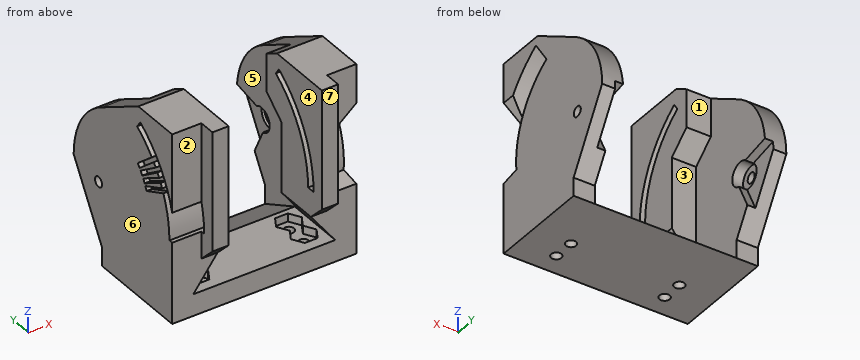
```python
from build123d import *

# Parameters (mm, degrees)
CROQUIS1_W              = 34
CROQUIS1_H              = 19
SALIENTE_EXTRUIR1_DEPTH = 35
CROQUIS2_W              = 26.2
CROQUIS2_H              = 31
CORTAR_EXTRUIR1_DEPTH   = 25
CORTAR_EXTRUIR3_DEPTH   = 26.2
SALIENTE_EXTRUIR2_DEPTH = 34
CROQUIS10_W             = 26.2
CROQUIS10_H             = 25.966324345
CORTAR_EXTRUIR4_DEPTH   = 10
CROQUIS18_R             = 0.95
CORTAR_EXTRUIR11_DEPTH  = 4
CORTAR_EXTRUIR12_DEPTH  = 1.5
CORTAR_EXTRUIR14_START  = -34
CROQUIS21_R             = 0.95
CORTAR_EXTRUIR14_DEPTH  = 34
SALIENTE_EXTRUIR3_DEPTH = 8
CROQUIS25_W             = 3
CROQUIS25_H             = 25
SALIENTE_EXTRUIR4_DEPTH = 3
CROQUIS43_W             = 4.5
CROQUIS43_H             = 12
SALIENTE_EXTRUIR8_DEPTH = 4
CORTAR_EXTRUIR18_DEPTH  = 7.4
CORTAR_EXTRUIR16_START  = -34
CORTAR_EXTRUIR16_DEPTH  = 26.6
CORTAR_EXTRUIR20_START  = -1.5
CORTAR_EXTRUIR20_DEPTH  = 1.5
CORTAR_EXTRUIR21_DEPTH  = 27.7
CORTAR_EXTRUIR22_START  = -34
CORTAR_EXTRUIR22_DEPTH  = 34
CORTAR_EXTRUIR23_DEPTH  = 3
CROQUIS36_R             = 2.2
CORTAR_EXTRUIR24_DEPTH  = 2
CORTAR_EXTRUIR25_START  = 28.2
CROQUIS36_2_R           = 2.2
CORTAR_EXTRUIR25_DEPTH  = 28.2
CORTAR_EXTRUIR26_START  = -34
CORTAR_EXTRUIR26_DEPTH  = 34
CORTAR_EXTRUIR27_DEPTH  = 1
CORTAR_EXTRUIR28_START  = -23.2
CORTAR_EXTRUIR28_DEPTH  = 23.2
CORTAR_EXTRUIR29_DEPTH  = 26.2


with BuildPart() as part:
    # Croquis1 → Saliente-Extruir1 (new body)
    with BuildSketch(Plane.XY):
        with Locations((-31.887263086, 5.12254902)):
            Rectangle(CROQUIS1_W, CROQUIS1_H)
    extrude(amount=SALIENTE_EXTRUIR1_DEPTH)

    # Croquis2 → Cortar-Extruir1 (cut)
    with BuildSketch(Plane.XZ.offset(4.37745098)):
        with Locations((-31.887263086, 19.5)):
            Rectangle(CROQUIS2_W, CROQUIS2_H)
    extrude(amount=-CORTAR_EXTRUIR1_DEPTH, mode=Mode.SUBTRACT)

    # Croquis4 → Cortar-Extruir3 (cut)
    with BuildSketch(Plane.ZY.offset(18.787263086)):
        Polygon((4, 14.62254902), (4, 6.62254902), (0, 14.62254902), align=None)
    extrude(amount=CORTAR_EXTRUIR3_DEPTH, mode=Mode.SUBTRACT)

    # Croquis9 → Saliente-Extruir2 (add)
    with BuildSketch(Plane(origin=(-14.887263086, 0, 0), x_dir=(0, 0, -1), z_dir=(1, 0, 0))):
        with BuildLine():
            Line((-29.315831827, 14.62254902), (-3.349507482, 14.62254902))
            ThreePointArc((-3.349507482, 14.62254902), (-16.332669655, 22.37254902), (-29.315831827, 14.62254902))
        make_face()
    extrude(amount=-SALIENTE_EXTRUIR2_DEPTH)

    # Croquis10 → Cortar-Extruir4 (cut)
    with BuildSketch(Plane.XZ.offset(-14.62254902)):
        with Locations((-31.887263086, 16.332669655)):
            Rectangle(CROQUIS10_W, CROQUIS10_H)
    extrude(amount=-CORTAR_EXTRUIR4_DEPTH, mode=Mode.SUBTRACT)

    # Croquis18 → Cortar-Extruir11 (cut)
    with BuildSketch(Plane(origin=(0, 0, 0), x_dir=(-1, 0, 0), z_dir=(0, 0, -1))):
        with Locations((41.887263086, -0.37745098)):
            Circle(CROQUIS18_R)
        with Locations((21.887263086, -0.37745098)):
            Circle(CROQUIS18_R)
        with Locations((21.887263086, 3.62254902)):
            Circle(CROQUIS18_R)
        with Locations((41.887263086, 3.62254902)):
            Circle(CROQUIS18_R)
    extrude(amount=-CORTAR_EXTRUIR11_DEPTH, mode=Mode.SUBTRACT)

    # Croquis19 → Cortar-Extruir12 (cut)
    with BuildSketch(Plane.XY.offset(4)):
        Polygon((-39.520126982, -0.37745098), (-40.67482752, 1.62254902), (-39.520126982, 3.62254902), (-40.703695034, 5.67254902), (-43.070831137, 5.67254902), (-44.254399189, 3.62254902), (-43.099698651, 1.62254902), (-44.254399189, -0.37745098), (-43.070831137, -2.42745098), (-40.703695034, -2.42745098), align=None)
        Polygon((-19.520126982, -0.37745098), (-20.67482752, 1.62254902), (-19.520126982, 3.62254902), (-20.703695034, 5.67254902), (-23.070831137, 5.67254902), (-24.254399189, 3.62254902), (-23.099698651, 1.62254902), (-24.254399189, -0.37745098), (-23.070831137, -2.42745098), (-20.703695034, -2.42745098), align=None)
    extrude(amount=-CORTAR_EXTRUIR12_DEPTH, mode=Mode.SUBTRACT)

    # Croquis21 → Cortar-Extruir14 (cut)
    with BuildSketch(Plane(origin=(-14.887263086, 0, 0), x_dir=(0, 0, -1), z_dir=(1, 0, 0)).offset(CORTAR_EXTRUIR14_START)):
        with Locations((-15, 15.62254902)):
            Circle(CROQUIS21_R)
    extrude(amount=CORTAR_EXTRUIR14_DEPTH, mode=Mode.SUBTRACT)

    # Croquis23 → Saliente-Extruir3 (add)
    with BuildSketch(Plane.XZ.offset(4.37745098)):
        Polygon((-44.987263086, 35), (-40.487263086, 35), (-40.487263086, 10), (-44.987263086, 4), align=None)
        Polygon((-18.787263086, 35), (-23.287263086, 35), (-23.287263086, 10), (-18.787263086, 4), align=None)
    extrude(amount=-SALIENTE_EXTRUIR3_DEPTH)

    # Croquis25 → Saliente-Extruir4 (add)
    with BuildSketch(Plane.XZ.offset(4.37745098)):
        with Locations((-41.987263086, 22.5)):
            Rectangle(CROQUIS25_W, CROQUIS25_H)
        with Locations((-21.787263086, 22.5)):
            Rectangle(CROQUIS25_W, CROQUIS25_H)
    extrude(amount=SALIENTE_EXTRUIR4_DEPTH)

    # Croquis43 → Saliente-Extruir8 (add)
    with BuildSketch(Plane(origin=(0, 3.62254902, 0), x_dir=(1, 0, 0), z_dir=(0, 1, 0))):
        with Locations((-21.037263086, -29)):
            Rectangle(CROQUIS43_W, CROQUIS43_H)
        with Locations((-42.737263086, -29)):
            Rectangle(CROQUIS43_W, CROQUIS43_H)
    extrude(amount=SALIENTE_EXTRUIR8_DEPTH)

    # Croquis27 → Cortar-Extruir18 (cut)
    with BuildSketch(Plane(origin=(-14.887263086, 0, 0), x_dir=(0, 0, -1), z_dir=(1, 0, 0))):
        with BuildLine():
            Line((-13.549434023, -0.942577786), (-12.635457129, -5.887329478))
            ThreePointArc((-12.635457129, -5.887329478), (-24.560215782, -3.790544761), (-33.492032026, 4.383746258))
            Line((-33.492032026, 4.383746258), (-29.371216121, 7.25740019))
            ThreePointArc((-29.371216121, 7.25740019), (-22.651516826, 0.859017666), (-13.549434023, -0.942577786))
        make_face()
    extrude(amount=-CORTAR_EXTRUIR18_DEPTH, mode=Mode.SUBTRACT)

    # Croquis24 → Cortar-Extruir16 (cut)
    with BuildSketch(Plane(origin=(-14.887263086, 0, 0), x_dir=(0, 0, -1), z_dir=(1, 0, 0)).offset(CORTAR_EXTRUIR16_START)):
        with BuildLine():
            Line((-15, -3.62745098), (-15, -5.12726591))
            ThreePointArc((-15, -5.12726591), (-24.876851848, -2.625810281), (-32.372332418, 4.275439874))
            Line((-32.372332418, 4.275439874), (-31.142668885, 5.135569413))
            ThreePointArc((-31.142668885, 5.135569413), (-24.183902835, -1.295442254), (-15, -3.62745098))
        make_face()
    extrude(amount=CORTAR_EXTRUIR16_DEPTH, mode=Mode.SUBTRACT)

    # Croquis29 → Cortar-Extruir20 (cut)
    with BuildSketch(Plane.ZY.offset(18.787263086).offset(CORTAR_EXTRUIR20_START)):
        with BuildLine():
            Line((17.797402962, 22.299641931), (16.5, 15.62254902))
            ThreePointArc((16.5, 15.62254902), (15.426958984, 14.184596995), (13.743058632, 14.803953638))
            Line((13.743058632, 14.803953638), (6.296886003, 18.432060872))
            ThreePointArc((6.296886003, 18.432060872), (11.631045274, 21.603150873), (17.797402962, 22.299641931))
        make_face()
    extrude(amount=CORTAR_EXTRUIR20_DEPTH, mode=Mode.SUBTRACT)

    # Croquis29<2> → Cortar-Extruir21 (cut)
    with BuildSketch(Plane.ZY.offset(18.787263086)):
        with BuildLine():
            Line((17.797402962, 22.299641931), (16.5, 15.62254902))
            ThreePointArc((16.5, 15.62254902), (15.426958984, 14.184596995), (13.743058632, 14.803953638))
            Line((13.743058632, 14.803953638), (6.296886003, 18.432060872))
            ThreePointArc((6.296886003, 18.432060872), (11.631045274, 21.603150873), (17.797402962, 22.299641931))
        make_face()
    extrude(amount=CORTAR_EXTRUIR21_DEPTH, mode=Mode.SUBTRACT)

    # Croquis30 → Cortar-Extruir22 (cut)
    with BuildSketch(Plane.ZY.offset(48.887263086).offset(CORTAR_EXTRUIR22_START)):
        Polygon((29.315831827, 14.62254902), (35, 4.827802707), (35, 14.62254902), align=None)
    extrude(amount=CORTAR_EXTRUIR22_DEPTH, mode=Mode.SUBTRACT)

    # Croquis35 → Cortar-Extruir23 (cut)
    with BuildSketch(Plane.XZ.offset(4.37745098)):
        Polygon((-20.287263086, 23.262320252), (-14.887263086, 23.262320252), (-14.887263086, 27.796275801), align=None)
    extrude(amount=-CORTAR_EXTRUIR23_DEPTH, mode=Mode.SUBTRACT)

    # Croquis36 → Cortar-Extruir24 (cut)
    with BuildSketch(Plane.ZY.offset(18.787263086)):
        with Locations((15, 15.62254902)):
            Circle(CROQUIS36_R)
    extrude(amount=-CORTAR_EXTRUIR24_DEPTH, mode=Mode.SUBTRACT)

    # Croquis36<2> → Cortar-Extruir25 (cut)
    with BuildSketch(Plane.ZY.offset(18.787263086).offset(CORTAR_EXTRUIR25_START)):
        with Locations((15, 15.62254902)):
            Circle(CROQUIS36_2_R)
    extrude(amount=-CORTAR_EXTRUIR25_DEPTH, mode=Mode.SUBTRACT)

    # Croquis38 → Cortar-Extruir26 (cut)
    with BuildSketch(Plane.ZY.offset(48.887263086).offset(CORTAR_EXTRUIR26_START)):
        Polygon((3.349507482, 14.62254902), (16.332669655, 22.37254902), (3.349507482, 22.37254902), align=None)
    extrude(amount=CORTAR_EXTRUIR26_DEPTH, mode=Mode.SUBTRACT)

    # Croquis40 → Cortar-Extruir27 (cut)
    with BuildSketch(Plane.ZY.offset(48.887263086)):
        Polygon((24.462469518, 4.967906508), (27.804965088, 0.984475403), (27.192129534, 0.470245316), (23.849633963, 4.45367642), align=None)
        Polygon((23.499956861, 4.180731289), (26.48255433, -0.078859342), (25.827232695, -0.537720491), (22.844635226, 3.72187014), align=None)
        Polygon((22.469633136, 3.484764914), (25.069633136, -1.018567186), (24.376812813, -1.418567186), (21.776812813, 3.084764914), align=None)
        Polygon((21.381853505, 2.883100647), (23.579468466, -1.829699846), (22.854422236, -2.167794455), (20.656807275, 2.545006037), align=None)
    extrude(amount=-CORTAR_EXTRUIR27_DEPTH, mode=Mode.SUBTRACT)

    # Croquis41 → Cortar-Extruir28 (cut)
    with BuildSketch(Plane(origin=(-20.287263086, 0, 0), x_dir=(0, 0, -1), z_dir=(1, 0, 0)).offset(CORTAR_EXTRUIR28_START)):
        Polygon((-10, -4.37745098), (-10, -7.37745098), (-13, -7.37745098), align=None)
    extrude(amount=CORTAR_EXTRUIR28_DEPTH, mode=Mode.SUBTRACT)

    # Croquis44 → Cortar-Extruir29 (cut)
    with BuildSketch(Plane.ZY.offset(18.787263086)):
        Polygon((23, 7.62254902), (26.362551066, 7.62254902), (23, 3.62254902), align=None)
    extrude(amount=CORTAR_EXTRUIR29_DEPTH, mode=Mode.SUBTRACT)


solid = part.part
```
Source: CAD feature listing. Evaluate the final solid. Frame: model axes, mm. Face numbers are marked on the shaded views. A direction names the side the tool comes from. Round coordinates to 2 decimals unless told otherwise and drop trailing zeros. Write each loop counter-clockwise with the first axis right and the second up, starting at its lowest first coordinate (ties: lowest second). Pieces come first, ordered by that corner, then holes. Notation, with made-up numbers: M 4,21 L 30,21 A12 ccw 30,37 Z; hole C 63.5,45 d2. An arc over 180 degrees is marked long. Answer as a JSON object with one key per item and string values. Group by question number.
(1) Section query B-B on x = -33. Output: boundary loops of the cut face in (y, z).
(2) Reachability of the marked faces 1, 2, 3 and 4 from +Z, -Z, +X, -X, +Y, -Y: full face, straight path, thin tool, end or side. Return the list, or none.
(3) Mould query, pull axis X, two halves, no side actions, for the marked faces 5, 6 and 7. Classes: +X half, -X half, draft (parallel to the pull), parting line (faces both ways), or undercut.
(4) First-contact query: pin 1 (3 mm diameter, centred on x = -30, y = 5.5, fed in from +Z); pin 2 (1.3 mm diameter, centred on x = -20, z = 29.5, fed in from +Y); pin 3 (1.2 mm diameter, centred on x = -21.5, z = 3.5, fed in from -Y). Flat tips, straight axial feed; report the tip coordinate or a pass-through.
(5) Section query A-A on z = 11.5. Output: boundary loops of the cut face in (x, y), then the cut area to 3 significant figures.
(6) Ray query, line 1 (X direction, y = -4, z = 12.5); line 2 (X direction, y = 9.75, z = 20.5); line 3 (Y direction, x = -30.5, z = 3.5). Return the intervals inside material, ascending. Write a range as [from, to].
Computed values:
{
 "1": {"outline": "M -4.38,0 L 14.62,0 L 6.62,4 L -4.38,4 Z"},
 "2": {"face 1": "+Z, +Y", "face 2": "+Z, -Z, -X, -Y", "face 3": "+Y", "face 4": "+Z, +Y, -Y"},
 "3": {"face 5": "undercut", "face 6": "-X half", "face 7": "draft"},
 "4": {"pin 1": "z = 4", "pin 2": "y = 7.62", "pin 3": "y = -4.38"},
 "5": {"outline": "M -48.89,-4.38 L -43.49,-4.38 L -43.49,-5.88 L -40.49,-5.88 L -40.49,3.62 L -44.99,3.62 L -44.99,15.9 L -46.49,15.9 L -46.49,19.49 L -48.89,19.49 Z; M -23.29,-5.88 L -20.29,-5.88 L -20.29,-4.38 L -14.89,-4.38 L -14.89,19.49 L -17.29,19.49 L -17.29,15.9 L -18.79,15.9 L -18.79,3.62 L -23.29,3.62 Z", "area": "256 mm^2"},
 "6": {"line 1": "[-48.89, -40.49], [-23.29, -14.89]", "line 2": "[-48.89, -44.99], [-18.79, -14.89]", "line 3": "[-4.38, 7.62]"}
}
